CAD build for the part. Positions are in the model's coordinates, mm. Round coordinates to 2 decimals unless told otherwise and drop trailing zeros. Order: outer loops, then holes, each group sorted by start corner. A loop starts at its lowest first (then second) coordinate and runs counter-clockwise, first axis right, second up. Notation, with made-up numbers: M 27.5,-6.75 L 51.5,-6.75 A21 cw 51.5,15.25 Z; hole C 89,-40 d4. An arc over 180 degrees is marked long. Answer as a JSON object with one key per item and string values.
```python
from build123d import *

# Parameters (mm, degrees)
SKETCH_1_W          = 50
SKETCH_1_H          = 50
EXTRUDE_1_DEPTH     = 10
FILLET_1_R          = 20
FILLET_2_R          = 1
SKETCH_3_R          = 4
CUT_EXTRUDE_2_DEPTH = 10
SKETCH_4_R          = 1.65
CUT_EXTRUDE_3_DEPTH = 10
CUT_EXTRUDE_4_DEPTH = 10


with BuildPart() as part:
    # 草图1 → 凸台-拉伸1 (new body)
    with BuildSketch(Plane.XY):
        Rectangle(SKETCH_1_W, SKETCH_1_H)
    extrude(amount=EXTRUDE_1_DEPTH)

    # 圆角1
    fillet_1_edges = [part.edges().sort_by_distance(p)[0] for p in [
        (25, -25, 5),
        (25, 25, 5),
    ]]
    fillet(fillet_1_edges, radius=FILLET_1_R)

    # 圆角2
    fillet_2_edges = [part.edges().sort_by_distance(p)[0] for p in [
        (-25, 0, 10),
        (25, 0, 0),
        (25, 0, 10),
        (-10, -25, 10),
        (-10, 25, 0),
        (19.142135624, 19.142135624, 0),
        (19.142135624, -19.142135624, 0),
        (-10, 25, 10),
        (19.142135624, 19.142135624, 10),
        (19.142135624, -19.142135624, 10),
        (-10, -25, 0),
        (-25, 0, 0),
        (-25, -25, 5),
        (-25, 25, 5),
    ]]
    fillet(fillet_2_edges, radius=FILLET_2_R)

    # 草图3 → 切除-拉伸2 (cut)
    with BuildSketch(Plane.XY.offset(10)):
        with Locations((-10, 10)):
            Circle(SKETCH_3_R)
        with Locations(Location((10, 10, 0), (0, 0, 180))):
            Circle(SKETCH_3_R)
        with Locations((10, -10)):
            Circle(SKETCH_3_R)
        with Locations(Location((-10, -10, 0), (0, 0, 180))):
            Circle(SKETCH_3_R)
    extrude(amount=-CUT_EXTRUDE_2_DEPTH, mode=Mode.SUBTRACT)

    # 草图4 → 切除-拉伸3 (cut)
    with BuildSketch(Plane.XY.offset(10)):
        with Locations((-20, -10)):
            Circle(SKETCH_4_R)
        with Locations((-20, 10)):
            Circle(SKETCH_4_R)
        with Locations((-12, 18)):
            Circle(SKETCH_4_R)
        with Locations((8, 18)):
            Circle(SKETCH_4_R)
    extrude(amount=-CUT_EXTRUDE_3_DEPTH, mode=Mode.SUBTRACT)

    # 草图5 → 切除-拉伸4 (cut)
    with BuildSketch(Plane.XY.offset(10)):
        with BuildLine():
            Line((-25, 10), (-25, 6.241461477))
            Line((-25, 6.241461477), (-27.089820729, 25))
            Line((-27.089820729, 25), (-10, 25))
            ThreePointArc((-10, 25), (-20.606601718, 20.606601718), (-25, 10))
        make_face()
    extrude(amount=-CUT_EXTRUDE_4_DEPTH, mode=Mode.SUBTRACT)


solid = part.part
```
Item 1: Saw through at A-A on z = 5.25. State how many separate pieces and enclosed holes the cut face has, and give its area (3 significant figures).
Worked answers:
{"separate pieces": "1", "enclosed holes": "8", "area": "2,040 mm2"}
Item 2: Drop flat-ended pins along their axis: pin 1 Ø2 at (y, z) = (11.5, 6.5) entering from -X; pin 2 Ø1.5 at (y, z) = (-6, 2) entering from +X; pin 3 Ø5 at (y, z) = (17, 5) entering from +X. Give the stop position or say it passes through.
Worked answers:
{"pin 1": "stops at x = -24.99", "pin 2": "stops at x = 25", "pin 3": "stops at x = 22.6"}
Item 3: Wall check: line 1 along Y through (x, z) = (-10, 7.5); line 2 along Y through (x, z) = (9, 4.5); line 3 along X through (y, z) = (-13, 4.25). Give the ranges that are in metal, low to high. Write a range as [from, to].
Worked answers:
{"line 1": "y = [-25, -14], [-6, 6], [14, 25]", "line 2": "y = [-24.6, -13.87], [-6.13, 6.13], [13.87, 16.69], [19.31, 24.6]", "line 3": "x = [-25, -12.65], [-7.35, 7.35], [12.65, 23.33]"}
Item 4: Saw through at B-B on x = -21. List the corners of the cut face in (y, z), and give its area (3 significant figures).
Worked answers:
{"outline": "M -25,1 A1 ccw -24,0 L -11.31,0 L -11.31,10 L -24,10 A1 ccw -25,9 Z; M -8.69,0 L 8.69,0 L 8.69,10 L -8.69,10 Z; M 11.31,0 L 20.2,0 L 20.2,10 L 11.31,10 Z", "area": "399 mm2"}
Item 5: Two-plate mould, pull along X, no slides. Class faces 1 (the flat face through (25, 0, 5)), 2 (the flat face through (0, 0, 0)), 3 (the cylindrical face through (7.785, 19.636, 5.07)): released by +X, released by -X, zero draft, split by the parting line, or undercut.
Worked answers:
{"face 1": "released by +X", "face 2": "zero draft", "face 3": "undercut"}
